Design review of the part built by this model. Coordinates are the model's own, in mm. Coordinates: 2 decimals unless noted, no trailing zeros. Loops run counter-clockwise (first coordinate to the right, second up) from the corner with the lowest first, then second, coordinate; pieces in that order, holes last.
Q1. Draft analysis for pull direction Z (two halves, no side actions). For faces 1 (the face through (1.73, 2.32, 7.81)), 2 (the face through (3, 90, 10)), 3 (the face through (2.17, 4.68, -9.76)), state which applies: released by +Z, released by -Z, zero draft, split by the parting line, or undercut.
Q2. For P1, Ø0.6, axis at x = 0, z = 0, coming from the +Y side; P2, Ø1, axis at x = -7.5, y = 55, coming from the -Z side; P3, Ø6, axis at x = -2.5, y = 26.5, coming from the -Z side, all flat-tipped, find the tip position at first contact; note any pin that passes through.
Q3. Wall thickness on probe 1 along Z at (x, y) = (0, 41); probe 2 along Y at (x, z) = (-10, 2.5); probe 3 along Z at (x, y) = (-3.5, 71): over which ranges is each line inside the solid? List them lowest first.
Q4. Add section A-A on y = 49. Give the boundary of the cut face in (x, z), and give its area (3 significant figures).
Autodesk Inventor part; units mm, degrees
ref_plane "YZ Plane" through (0, 0, 0) normal (1, 0, 0) x (0, 1, 0)
ref_plane "XZ Plane" through (0, 0, 0) normal (0, 1, 0) x (-1, 0, 0)
ref_plane "XY Plane" through (0, 0, 0) normal (0, 0, 1) x (1, 0, 0)
sketch "Szkic1" plane through (0, 0, 0) normal (0, 0, 1) x (1, 0, 0)
  line L0 (1, -90) -> (-1, -90)
  line L1 (-10, -81) -> (-10, 90)
  line L2 (-10, 90) -> (-10, 90)
  line L3 (10, 90) -> (10, -81)
  line L4 (10, -90) -> (-10, 90) construction
  line L5 (-10, -90) -> (10, 90) construction
  arc A0 (1, -90) -> (10, -81) centre (1, -81) ccw
  arc A1 (-10, -81) -> (-1, -90) centre (-1, -81) ccw
  line L6 (-10, 90) -> (-14, 90)
  line L7 (-15, 89) -> (-15, 89)
  line L8 (-14, 88) -> (-10, 88)
  line L9 (-10, 88) -> (-10, 90)
  line L10 (10, 90) -> (14, 90)
  line L11 (15, 89) -> (15, 89)
  line L12 (14, 88) -> (10, 88)
  line L13 (10, 88) -> (10, 90)
  arc A2 (14, 88) -> (15, 89) centre (14, 89) ccw
  arc A3 (15, 89) -> (14, 90) centre (14, 89) ccw
  arc A4 (-15, 89) -> (-14, 88) centre (-14, 89) ccw
  arc A5 (-14, 90) -> (-15, 89) centre (-14, 89) ccw
  line L14 (-8, 88) -> (-8, -81)
  arc A6 (-8, -81) -> (-1, -88) centre (-1, -81) ccw
  line L15 (-1, -88) -> (1, -88)
  arc A7 (1, -88) -> (8, -81) centre (1, -81) ccw
  line L16 (8, -81) -> (8, 88)
  arc A8 (-8, 88) -> (-10, 90) centre (-10, 88) ccw
  line L17 (10, 90) -> (10, 90)
  arc A9 (10, 90) -> (8, 88) centre (10, 88) ccw
  line L18 (0, -90) -> (0, 71.327) construction
  line L19 (0, -90) -> (0, -88)
  point P0 (0, 0)
  point P1 (-15, 88)
  point P2 (-15, 90)
  point P3 (15, 88)
  point P4 (-10, 90)
  point P5 (-10, 88)
  dimension "d0" = 20
  dimension "d1" = 180
  dimension "d2" = 9
  dimension "d3" = 9
  dimension "d4" = 5
  dimension "d5" = 2
  dimension "d6" = 5
  dimension "d7" = 1
  dimension "d8" = 1
  dimension "d9" = 1
  dimension "d10" = 1
  dimension "d11" = 2
  dimension "d12" = 2
  dimension "d13" = 2
revolve "Obrót1" add sketch "Szkic1" angle 360 about axis through (0, -90, 0) along (0, 1, 0) contours L0 A1 L1 A8 L14 A6 L15 L19 | L8 A4 A5 L6 L1
properties part number "fiolka" material "Szkło"
Entries:
1. face 1: undercut
1. face 2: zero draft
1. face 3: split by the parting line
2. P1: stops at y = -88
2. P2: stops at z = -7.14
2. P3: stops at z = -10
3. probe 1: z = -10 to -8, 8 to 10
3. probe 2: y = 88 to 90
3. probe 3: z = -9.37 to -7.19, 7.19 to 9.37
4. outline: circle Ø20 at (0, 0); hole circle Ø16 at (0, 0)
4. area: 113 mm2
